Build history of the part. All positions in model axes, mm. A direction names the side the tool comes from. Round coordinates to 2 decimals unless told otherwise and drop trailing zeros. Write each loop counter-clockwise with the first axis right and the second up, starting at its lowest first coordinate (ties: lowest second). Pieces come first, ordered by that corner, then holes. Notation, with made-up numbers: M 47.25,5.5 L 62.25,5.5 A25 cw 62.25,44.5 Z; hole C 40,62 d5. An arc over 180 degrees is marked long. Write item = value, one per line.
from build123d import *

# Parameters (mm, degrees)
SKETCH1_R             = 5
SKETCH1_R_2           = 3
BOSS_EXTRUDE1_DEPTH   = 4
SKETCH1_R_3           = 1
BOSS_EXTRUDE1_2_DEPTH = 4
SKETCH2_R             = 4
BOSS_EXTRUDE2_DEPTH   = 8
SKETCH3_W             = 0.5
SKETCH3_H             = 2.4979992
BOSS_EXTRUDE3_DEPTH   = 4


with BuildPart() as part:
    # Sketch1 → Boss-Extrude1 (new body)
    with BuildSketch(Plane.XY):
        Circle(SKETCH1_R)
        Circle(SKETCH1_R_2, mode=Mode.SUBTRACT)
    extrude(amount=-BOSS_EXTRUDE1_DEPTH)



with BuildPart() as body_2:
    # Sketch1 → Boss-Extrude1 2 (new body)
    with BuildSketch(Plane.XY):
        Circle(SKETCH1_R_3)
    extrude(amount=-BOSS_EXTRUDE1_2_DEPTH)


with BuildPart() as part_1:
    add(part.part)

    add(body_2.part)  # Boss-Extrude2 merges body 2
    # Sketch2 → Boss-Extrude2 (add)
    with BuildSketch(Plane(origin=(0, 0, -4), x_dir=(-1, 0, 0), z_dir=(0, 0, -1))):
        Circle(SKETCH2_R)
    extrude(amount=BOSS_EXTRUDE2_DEPTH)

    # Sketch3 → Boss-Extrude3 (add)
    with BuildSketch(Plane(origin=(0, 0, -12), x_dir=(-1, 0, 0), z_dir=(0, 0, -1))):
        with Locations((-3.55, 0)):
            Rectangle(SKETCH3_W, SKETCH3_H)
        with Locations((3.55, 0)):
            Rectangle(SKETCH3_W, SKETCH3_H)
    extrude(amount=BOSS_EXTRUDE3_DEPTH)


solid = part_1.part
1. Band-saw the part on B-B (x = 0). List the corners of the cut face in (y, z).
Responses:
outline = M -5,-4 L -4,-4 L -4,-12 L 4,-12 L 4,-4 L 5,-4 L 5,0 L 3,0 L 3,-4 L 1,-4 L 1,0 L -1,0 L -1,-4 L -3,-4 L -3,0 L -5,0 Z
2. Mould opens along X. For faces 6 (the face through (-3.8, 0, -14)), 7 (the face through (1, 1, -4)), 8 (the face through (-0.1, -3.3, 0)) say: pulls with the +X half, pulls with the -X half, needs draft (parallel to the pull), parting line crosses it, or undercut.
Responses:
face_6 = pulls with the -X half
face_7 = undercut
face_8 = needs draft
3. Probe probe 1 along Y at (x, z) = (0, -2); probe 2 along Z at (x, y) = (2.75, -1.5); probe 3 along Z at (x, y) = (3, -3.25). List the from-to ranges inside material, lowest first.
Responses:
probe_1 = -5 to -3, -1 to 1, 3 to 5
probe_2 = -12 to 0
probe_3 = -4 to 0
4. Tool access for faces 1 (the face through (3.3, 0, -14)), 2 (the face through (0.867, -3.905, -7.944)), 3 (the face through (-1.08, -4.88, -1.97)), 4 (the face through (-3, 0, -2)), 5 (the face through (3.8, 0, -14)): list every direction of +Z, -Z, +X, -X, +Y, -Y with a clear straight run to the whole face (end or side of a thin tool).
Responses:
face_1 = -Z, +Y, -Y
face_2 = -Z
face_3 = +Z, -Z
face_4 = +Z
face_5 = -Z, +X, +Y, -Y
5. Band-saw the part on C-C (z = -9.25). List the corners of the cut face in (x, y), plus the area to 3 significant figures.
Responses:
outline = C 0,0 d8
area = 50.3 mm²
6. Band-saw the part on D-D (x = 1.5). List the corners of the cut face in (y, z).
Responses:
outline = M -4.77,-4 L -3.71,-4 L -3.71,-12 L 3.71,-12 L 3.71,-4 L 4.77,-4 L 4.77,0 L 2.6,0 L 2.6,-4 L -2.6,-4 L -2.6,0 L -4.77,0 Z
7. Flat gauge pins, fed straight in: pin 1 (2 mm diameter, centred on x = -4, z = -6.5, fed in from +Y); pin 2 (2 mm diameter, centred on y = -0.5, z = -14, fed in from -X); pin 3 (1 mm diameter, centred on x = -1.5, y = 1, fed in from +Z). Where does each tip first touch, or does it go through?
Responses:
pin_1 = 2.65
pin_2 = -3.8
pin_3 = -4
8. Band-saw the part on A-A (y = 0). List the corners of the cut face in (x, z).
Responses:
outline = M -5,-4 L -4,-4 L -4,-12 L -3.8,-12 L -3.8,-16 L -3.3,-16 L -3.3,-12 L 3.3,-12 L 3.3,-16 L 3.8,-16 L 3.8,-12 L 4,-12 L 4,-4 L 5,-4 L 5,0 L 3,0 L 3,-4 L 1,-4 L 1,0 L -1,0 L -1,-4 L -3,-4 L -3,0 L -5,0 Z
